Part model, mm, in its own coordinate system. A direction names the side the tool comes from. Give positions to 0.01 mm unless a question says otherwise; leave off trailing zeros. Loops run counter-clockwise (first coordinate to the right, second up) from the corner with the lowest first, then second, coordinate; pieces in that order, holes last. Notation, with made-up numbers: (29.5, -37.75) -> (70.5, -37.75) arc R19 cw to (70.5, -31.75) -> close; hole circle Ø1 at (80, 6). An arc over 180 degrees is marked (long way). Write item = value, one per line.
from build123d import *

# Parameters (mm, degrees)
SKETCH1_W           = 84.6
SKETCH1_H           = 63.2
SKETCH1_W_2         = 80.6
SKETCH1_H_2         = 59.2
BOSS_EXTRUDE1_DEPTH = 1
SKETCH2_W           = 82.6
SKETCH2_H           = 61.2
SKETCH2_W_2         = 80.6
SKETCH2_H_2         = 59.2
BOSS_EXTRUDE2_DEPTH = 2.5
SKETCH3_W           = 82.6
SKETCH3_H           = 61.2
SKETCH3_W_2         = 71.1
SKETCH3_H_2         = 53
BOSS_EXTRUDE3_DEPTH = 1
CHAMFER1_SIZE       = 2
CHAMFER1_SIZE_2     = 1
CHAMFER2_SIZE       = 0.5


with BuildPart() as part:
    # Sketch1 → Boss-Extrude1 (new body)
    with BuildSketch(Plane(origin=(0, 0, 0), x_dir=(1, 0, 0), z_dir=(0, 1, 0))):
        with Locations((42.3, 31.6)):
            Rectangle(SKETCH1_W, SKETCH1_H)
        with Locations((42.3, 31.6)):
            Rectangle(SKETCH1_W_2, SKETCH1_H_2, mode=Mode.SUBTRACT)
    extrude(amount=BOSS_EXTRUDE1_DEPTH)

    # Sketch2 → Boss-Extrude2 (add)
    with BuildSketch(Plane(origin=(0, 1, 0), x_dir=(1, 0, 0), z_dir=(0, 1, 0))):
        with Locations((42.3, 31.6)):
            Rectangle(SKETCH2_W, SKETCH2_H)
        with Locations((42.3, 31.6)):
            Rectangle(SKETCH2_W_2, SKETCH2_H_2, mode=Mode.SUBTRACT)
    extrude(amount=BOSS_EXTRUDE2_DEPTH)

    # Sketch3 → Boss-Extrude3 (add)
    with BuildSketch(Plane(origin=(0, 3.5, 0), x_dir=(1, 0, 0), z_dir=(0, 1, 0))):
        with Locations((42.3, 31.6)):
            Rectangle(SKETCH3_W, SKETCH3_H)
        with Locations((43.95, 31.6)):
            Rectangle(SKETCH3_W_2, SKETCH3_H_2, mode=Mode.SUBTRACT)
    extrude(amount=-BOSS_EXTRUDE3_DEPTH)

    # Chamfer1
    # the kernel refuses this chamfer: 2, 1 mm, written as the material it takes off along each edge
    with BuildSketch(Plane(origin=(79.5, 3.5, -58.1), x_dir=(0.9998508956747119, 0.01726807512366803, 0), z_dir=(0, 0, 1)), Plane(origin=(8.4, 3.5, -5.1), x_dir=(-0.9998508956747119, 0.01726807512366807, 0), z_dir=(0, 0, -1))) as chamfer1_piece_1:
        Polygon((CHAMFER1_SIZE * 0.999850895675, -CHAMFER1_SIZE * 0.0172680751237), (-CHAMFER1_SIZE_2 * 0.0172680751237, -CHAMFER1_SIZE_2 * 0.999850895675), (0, 0), align=None)
    extrude(amount=53, mode=Mode.SUBTRACT)
    with BuildSketch(Plane(origin=(79.5, 3.5, -5.1), x_dir=(0, 0.017268075123668084, 0.9998508956747119), z_dir=(-1, 0, 0)), Plane(origin=(8.4, 3.5, -58.1), x_dir=(0, 0.017268075123668087, -0.9998508956747116), z_dir=(1, 0, 0))) as chamfer1_piece_2:
        Polygon((CHAMFER1_SIZE * 0.999850895675, -CHAMFER1_SIZE * 0.0172680751237), (-CHAMFER1_SIZE_2 * 0.0172680751237, -CHAMFER1_SIZE_2 * 0.999850895675), (0, 0), align=None)
    extrude(amount=71.1, mode=Mode.SUBTRACT)
    with BuildSketch(Plane(origin=(8.4, 3.5, -58.1), x_dir=(0, 0.017268075123668087, -0.9998508956747116), z_dir=(1, 0, 0))) as chamfer1_piece_3a_section:
        Polygon((CHAMFER1_SIZE * 0.999850895675, -CHAMFER1_SIZE * 0.0172680751237), (-CHAMFER1_SIZE_2 * 0.0172680751237, -CHAMFER1_SIZE_2 * 0.999850895675), (0, 0), align=None)
    chamfer1_piece_3a = extrude(amount=76.279657748, mode=Mode.PRIVATE)
    chamfer1_piece_3a = split(chamfer1_piece_3a, bisect_by=Plane(origin=(79.5, 3.182784452, -58.774507016), z_dir=(1, 0, 0)), keep=Keep.TOP, mode=Mode.PRIVATE)
    with BuildSketch(Plane(origin=(79.5, 3.5, -63.279657748), x_dir=(0.9998508956747119, 0.01726807512366803, 0), z_dir=(0, 0, 1))) as chamfer1_piece_3b_section:
        Polygon((CHAMFER1_SIZE * 0.999850895675, -CHAMFER1_SIZE * 0.0172680751237), (-CHAMFER1_SIZE_2 * 0.0172680751237, -CHAMFER1_SIZE_2 * 0.999850895675), (0, 0), align=None)
    chamfer1_piece_3b = extrude(amount=58.179657748, mode=Mode.PRIVATE)
    chamfer1_piece_3b = split(chamfer1_piece_3b, bisect_by=Plane(origin=(80.174507016, 3.182784452, -58.1), z_dir=(0, 0, -1)), keep=Keep.TOP, mode=Mode.PRIVATE)
    chamfer1_piece_3 = chamfer1_piece_3a & chamfer1_piece_3b
    add(chamfer1_piece_3, mode=Mode.SUBTRACT)
    with BuildSketch(Plane(origin=(84.679657748, 3.5, -5.1), x_dir=(0, 0.017268075123668084, 0.9998508956747119), z_dir=(-1, 0, 0))) as chamfer1_piece_4a_section:
        Polygon((CHAMFER1_SIZE * 0.999850895675, -CHAMFER1_SIZE * 0.0172680751237), (-CHAMFER1_SIZE_2 * 0.0172680751237, -CHAMFER1_SIZE_2 * 0.999850895675), (0, 0), align=None)
    chamfer1_piece_4a = extrude(amount=76.279657748, mode=Mode.PRIVATE)
    chamfer1_piece_4a = split(chamfer1_piece_4a, bisect_by=Plane(origin=(79.5, 3.182784452, -4.425492984), z_dir=(1, 0, 0)), keep=Keep.TOP, mode=Mode.PRIVATE)
    with BuildSketch(Plane(origin=(79.5, 3.5, -58.1), x_dir=(0.9998508956747119, 0.01726807512366803, 0), z_dir=(0, 0, 1))) as chamfer1_piece_4b_section:
        Polygon((CHAMFER1_SIZE * 0.999850895675, -CHAMFER1_SIZE * 0.0172680751237), (-CHAMFER1_SIZE_2 * 0.0172680751237, -CHAMFER1_SIZE_2 * 0.999850895675), (0, 0), align=None)
    chamfer1_piece_4b = extrude(amount=58.179657748, mode=Mode.PRIVATE)
    chamfer1_piece_4b = split(chamfer1_piece_4b, bisect_by=Plane(origin=(80.174507016, 3.182784452, -5.1), z_dir=(0, 0, 1)), keep=Keep.TOP, mode=Mode.PRIVATE)
    chamfer1_piece_4 = chamfer1_piece_4a & chamfer1_piece_4b
    add(chamfer1_piece_4, mode=Mode.SUBTRACT)
    with BuildSketch(Plane(origin=(8.4, 3.5, 0.079657748), x_dir=(-0.9998508956747119, 0.017268075123668084, 0), z_dir=(0, 0, -1))) as chamfer1_piece_5a_section:
        Polygon((CHAMFER1_SIZE * 0.999850895675, -CHAMFER1_SIZE * 0.0172680751237), (-CHAMFER1_SIZE_2 * 0.0172680751237, -CHAMFER1_SIZE_2 * 0.999850895675), (0, 0), align=None)
    chamfer1_piece_5a = extrude(amount=58.179657748, mode=Mode.PRIVATE)
    chamfer1_piece_5a = split(chamfer1_piece_5a, bisect_by=Plane(origin=(7.725492984, 3.182784452, -5.1), z_dir=(0, 0, 1)), keep=Keep.TOP, mode=Mode.PRIVATE)
    with BuildSketch(Plane(origin=(79.5, 3.5, -5.1), x_dir=(0, 0.017268075123668084, 0.9998508956747119), z_dir=(-1, 0, 0))) as chamfer1_piece_5b_section:
        Polygon((CHAMFER1_SIZE * 0.999850895675, -CHAMFER1_SIZE * 0.0172680751237), (-CHAMFER1_SIZE_2 * 0.0172680751237, -CHAMFER1_SIZE_2 * 0.999850895675), (0, 0), align=None)
    chamfer1_piece_5b = extrude(amount=76.279657748, mode=Mode.PRIVATE)
    chamfer1_piece_5b = split(chamfer1_piece_5b, bisect_by=Plane(origin=(8.4, 3.182784452, -4.425492984), z_dir=(-1, 0, 0)), keep=Keep.TOP, mode=Mode.PRIVATE)
    chamfer1_piece_5 = chamfer1_piece_5a & chamfer1_piece_5b
    add(chamfer1_piece_5, mode=Mode.SUBTRACT)
    with BuildSketch(Plane(origin=(3.220342252, 3.5, -58.1), x_dir=(0, 0.017268075123668087, -0.9998508956747116), z_dir=(1, 0, 0))) as chamfer1_piece_6a_section:
        Polygon((CHAMFER1_SIZE * 0.999850895675, -CHAMFER1_SIZE * 0.0172680751237), (-CHAMFER1_SIZE_2 * 0.0172680751237, -CHAMFER1_SIZE_2 * 0.999850895675), (0, 0), align=None)
    chamfer1_piece_6a = extrude(amount=76.279657748, mode=Mode.PRIVATE)
    chamfer1_piece_6a = split(chamfer1_piece_6a, bisect_by=Plane(origin=(8.4, 3.182784452, -58.774507016), z_dir=(-1, 0, 0)), keep=Keep.TOP, mode=Mode.PRIVATE)
    with BuildSketch(Plane(origin=(8.4, 3.5, -5.1), x_dir=(-0.9998508956747119, 0.01726807512366807, 0), z_dir=(0, 0, -1))) as chamfer1_piece_6b_section:
        Polygon((CHAMFER1_SIZE * 0.999850895675, -CHAMFER1_SIZE * 0.0172680751237), (-CHAMFER1_SIZE_2 * 0.0172680751237, -CHAMFER1_SIZE_2 * 0.999850895675), (0, 0), align=None)
    chamfer1_piece_6b = extrude(amount=58.179657748, mode=Mode.PRIVATE)
    chamfer1_piece_6b = split(chamfer1_piece_6b, bisect_by=Plane(origin=(7.725492984, 3.182784452, -58.1), z_dir=(0, 0, -1)), keep=Keep.TOP, mode=Mode.PRIVATE)
    chamfer1_piece_6 = chamfer1_piece_6a & chamfer1_piece_6b
    add(chamfer1_piece_6, mode=Mode.SUBTRACT)

    # Chamfer2
    chamfer2_edges = [part.edges().sort_by_distance(p)[0] for p in [
        (1, 3.5, -31.6),
        (42.3, 3.5, -1),
        (83.6, 3.5, -31.6),
        (42.3, 3.5, -62.2),
    ]]
    chamfer(chamfer2_edges, length=CHAMFER2_SIZE)


solid = part.part
1) Drop flat-ended pins along their axis: P1, Ø1, axis at y = 2.5, z = -9.5, coming from the -X side; P2, Ø1, axis at x = 50, y = 2, coming from the +Z side; P3, Ø1.6, axis at y = 1.5, z = -22.5, coming from the +X side; P4, Ø8, axis at x = 45, z = -55, coming from the -Y side. Give the stop position or say it passes through.
Resolved:
P1 = 1
P2 = -1
P3 = 84.6
P4 = 2.5
2) Slice it at C-C, the plane y = 1.6. List the corners of the cut face in (x, z).
Resolved:
outline = (1, -62.2) -> (83.6, -62.2) -> (83.6, -1) -> (1, -1) -> close; hole (2, -61.2) -> (82.6, -61.2) -> (82.6, -2) -> (2, -2) -> close
3) Which spindle directions (+Z, -Z, +X, -X, +Y, -Y) get a long thin tool onto all of the face, cutting with end or side? Do faces 1 (the face through (42, 1, -61.2)), 2 (the face through (44.5, 3, -4.1)), 3 (the face through (42, 2, -62.2)), 4 (the face through (1, 2, -31)). Say none if no direction does.
Resolved:
face_1 = -Y
face_2 = +Y
face_3 = -Z, +X, -X, +Y
face_4 = +Z, -Z, -X, +Y
4) Slice it at A-A, the plane x = 56.5. List the corners of the cut face in (y, z), and give its area (4 significant figures).
Resolved:
outline = (0, -63.2) -> (1, -63.2) -> (1, -62.2) -> (3, -62.2) -> (3.5, -61.7) -> (3.5, -60.1) -> (2.5, -58.1) -> (2.5, -61.2) -> (0, -61.2) -> close; (0, -2) -> (2.5, -2) -> (2.5, -5.1) -> (3.5, -3.1) -> (3.5, -1.5) -> (3, -1) -> (1, -1) -> (1, 0) -> (0, 0) -> close
area = 12.95 mm²
5) Pull direction Z, two halves, no side cores. Call faces 5 (the face through (2, 1, -31)), 6 (the face through (39, 0, -1)), 7 (the face through (42, 2, -1)), 8 (the face through (42, 1, -2)): pulls with the +Z half, pulls with the -Z half, needs draft (parallel to the pull), parting line crosses it, or undercut.
Resolved:
face_5 = undercut
face_6 = needs draft
face_7 = pulls with the +Z half
face_8 = undercut
6) Slice it at B-B, the plane z = -17. List the corners of the cut face in (x, y).
Resolved:
outline = (0, 0) -> (2, 0) -> (2, 2.5) -> (8.4, 2.5) -> (6.4, 3.5) -> (1.5, 3.5) -> (1, 3) -> (1, 1) -> (0, 1) -> close; (79.5, 2.5) -> (82.6, 2.5) -> (82.6, 0) -> (84.6, 0) -> (84.6, 1) -> (83.6, 1) -> (83.6, 3) -> (83.1, 3.5) -> (81.5, 3.5) -> close
7) Drill centre lines: line 1 along X through (y, z) = (0.5, -41.5); line 2 along Z through (x, y) = (59, 0.4); line 3 along Z through (x, y) = (60, 1.55). Where is each one in solid material? Low to high. Write a range as [from, to].
Resolved:
line_1 = [0, 2], [82.6, 84.6]
line_2 = [-63.2, -61.2], [-2, 0]
line_3 = [-62.2, -61.2], [-2, -1]
